from build123d import *

# Parameters (mm, degrees)
F0_R     = 2.15265
F0_R_2   = 1.5
F0_R_3   = 5.969
F1_DEPTH = 3.175


with BuildPart() as f1:
    # F0 (on Top) → F1 (new body)
    with BuildSketch(Plane.XY):
        with BuildLine():
            ThreePointArc((18.600191, -18.161), (22.444669, -16.209442), (23.138398, -11.954172))
            Line((23.138398, -11.954172), (7.487077, 37.223663))
            ThreePointArc((7.487077, 37.223663), (3.361586, 40.970478), (-1.940047, 39.252633))
            Line((-1.940047, 39.252633), (-20.908597, 18.146535))
            ThreePointArc((-20.908597, 18.146535), (-21.775278, 16.764006), (-22.124412, 15.170071))
            Line((-22.124412, 15.170071), (-23.358191, -13.191519))
            ThreePointArc((-23.358191, -13.191519), (-22.040188, -16.692104), (-18.600191, -18.161))
            Line((-18.600191, -18.161), (18.600191, -18.161))
        make_face()
        with Locations((-18.600191, -13.3985)):
            Circle(F0_R, mode=Mode.SUBTRACT)
        with Locations((-7.62, -13.198227)):
            Circle(F0_R_2, mode=Mode.SUBTRACT)
        with Locations((-15.24, 0)):
            Circle(F0_R_2, mode=Mode.SUBTRACT)
        with Locations((7.62, -13.198227)):
            Circle(F0_R_2, mode=Mode.SUBTRACT)
        with Locations((18.600191, -13.3985)):
            Circle(F0_R, mode=Mode.SUBTRACT)
        with Locations((0, 7.366)):
            Circle(F0_R_3, mode=Mode.SUBTRACT)
        with Locations((15.24, 0)):
            Circle(F0_R_2, mode=Mode.SUBTRACT)
        with Locations((-17.366412, 14.963089)):
            Circle(F0_R, mode=Mode.SUBTRACT)
        with Locations((-7.62, 13.198227)):
            Circle(F0_R_2, mode=Mode.SUBTRACT)
        with Locations((7.62, 13.198227)):
            Circle(F0_R_2, mode=Mode.SUBTRACT)
        Polygon((6.161253, 35.538613), (4.176878, 32.101575), (0.208128, 32.101575), (-1.776247, 35.538613), (0.208128, 38.975652), (4.176878, 38.975652), align=None, mode=Mode.SUBTRACT)
    extrude(amount=F1_DEPTH)


solid = f1.part
The model under review builds one solid part; all positions refer to its coordinate system, in mm. A direction names the side the tool comes from. Round coordinates to 2 decimals unless told otherwise and drop trailing zeros. Order: outer loops, then holes, each group sorted by start corner. A loop starts at its lowest first (then second) coordinate and runs counter-clockwise, first axis right, second up. Notation, with made-up numbers: (51.25, 47.5) -> (86.25, 47.5) arc R23 cw to (86.25, 76.5) -> close; hole circle Ø11 at (19, 7). An arc over 180 degrees is marked (long way). Use CSV: the item, a comma, the result in double quotes. Start each with the question number.
(1) Consider section B-B on x = -4. Write out the cut boundary in (y, z) (3 decimals), and give its area (3 significant figures).
(2) Consider section A-A on y = 0. Write out the cut boundary in (x, z) (3 decimals).
(3) Consider section C-C on z = 1.4. State how many separate pieces and enclosed holes the cut face has, and give its area (3 significant figures).
(4) Tool access review of faces 1 (the face through (5.18, 33.84, 1.57)), 2 (the face through (-6, 12, 0)): name each direction out of +Z, -Z, +X, -X, +Y, -Y from which nothing blocks a thin tool from reaching the whole face with its end or side.
(5) Wall thickness on probe 1 along Y at (x, z) = (-16, 0.9); probe 2 along Y at (x, z) = (0, 1.7) (3 decimals); probe 3 along X at (y, z) = (-12, 2.95): over which ranges is each line inside the solid? List them lowest first. Write a range as from..to.
(6) Mouldability with a two-part tool opening along Y and no side actions: class faces 3 (the face through (0, -18.161, 2)), 4 (the face through (-6, 12, 3.175)), 5 (the face through (15.422, 12.291, 1.565)), 6 (the face through (2, 32.102, 2)) as pulls with the +Y half, pulls with the -Y half, needs draft (parallel to the pull), parting line crosses it, or undercut.
(7) Insertion check: pin 1 (1 mm diameter, centred on y = 19.5, z = 2, fed in from +X); pin 2 (1.5 mm diameter, centred on y = 14.5, z = 1.5, fed in from -X). Each pin has a flat end and moves straight along its axis. Give the tip position at first contact, or say it passes through.
(8) Consider section D-D on x = 19.5. Write out the cut boundary in (y, z) (3 decimals).
Responses:
1,outline,"(-18.161, 0) -> (2.936, 0) -> (2.936, 3.175) -> (-18.161, 3.175) -> close; (11.796, 0) -> (36.961, 0) -> (36.961, 3.175) -> (11.796, 3.175) -> close"
1,area,"147 mm²"
2,outline,"(-22.784, 0) -> (-16.74, 0) -> (-16.74, 3.175) -> (-22.784, 3.175) -> close; (-13.74, 0) -> (13.74, 0) -> (13.74, 3.175) -> (-13.74, 3.175) -> close; (16.74, 0) -> (19.334, 0) -> (19.334, 3.175) -> (16.74, 3.175) -> close"
3,separate pieces,"1"
3,enclosed holes,"11"
3,area,"1,740 mm²"
4,face 1,"+Z, -Z"
4,face 2,"-Z, +X, -X, +Y, -Y"
5,probe 1,"-18.16..-1.29, 1.29..13.3, 16.63..23.61"
5,probe 2,"-18.161..1.397, 13.335..32.462, 38.615..40.644"
5,probe 3,"-23.31..-20.24, -16.96..-8.52, -6.72..6.72, 8.52..16.96, 20.24..23.15"
6,face 3,"pulls with the -Y half"
6,face 4,"needs draft"
6,face 5,"pulls with the +Y half"
6,face 6,"undercut"
7,pin 1,"x = 13.29"
7,pin 2,"x = -22.19"
8,outline,"(-18.075, 0) -> (-15.354, 0) -> (-15.354, 3.175) -> (-18.075, 3.175) -> close; (-11.443, 0) -> (-0.522, 0) -> (-0.522, 3.175) -> (-11.443, 3.175) -> close"
